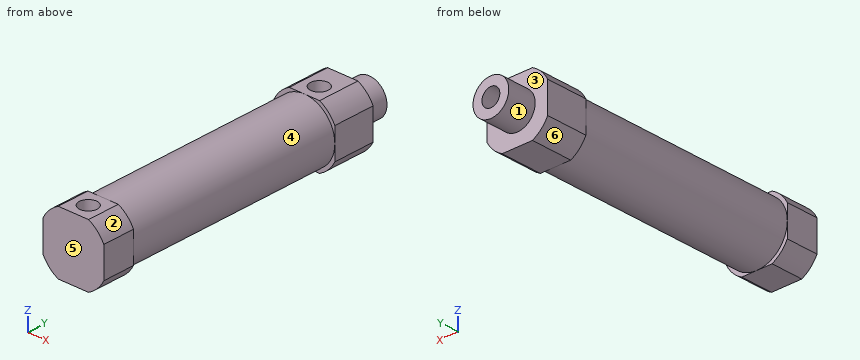
Autodesk Inventor part; units mm, degrees
ref_plane "YZ Plane" through (0, 0, 0) normal (1, 0, 0) x (0, 1, 0)
ref_plane "XZ Plane" through (0, 0, 0) normal (0, 1, 0) x (-1, 0, 0)
ref_plane "XY Plane" through (0, 0, 0) normal (0, 0, 1) x (1, 0, 0)
sketch "スケッチ1" plane through (0, 0, 0) normal (0, 1, 0) x (-1, 0, 0)
  circle A0 centre (0, 0) radius 8.5
  dimension "d0" = 17
extrude "押し出し1" add sketch "スケッチ1" along normal blind 61
sketch "スケッチ2" plane through (0, 61, 0) normal (0, 1, 0) x (1, 0, 0)
  circle A0 centre (0, 0) radius 9.5
  line L0 (8.5, -8.5) -> (-8.5, -8.5)
  line L1 (-8.5, -8.5) -> (-8.5, 8.5)
  line L2 (-8.5, 8.5) -> (8.5, 8.5)
  line L3 (8.5, 8.5) -> (8.5, -8.5)
  line L4 (8.5, -8.5) -> (-8.5, 8.5) construction
  line L5 (-8.5, -8.5) -> (8.5, 8.5) construction
  point P0 (8.5, -4.2426)
  point P1 (8.5, 4.2426)
  point P2 (4.2426, 8.5)
  point P3 (-4.2426, 8.5)
  point P4 (-8.5, 4.2426)
  point P5 (-8.5, -4.2426)
  point P6 (-4.2426, -8.5)
  point P7 (4.2426, -8.5)
  dimension "d3" = 19
  dimension "d4" = 17
  dimension "d5" = 17
extrude "押し出し2" add sketch "スケッチ2" along normal blind 11.6 contours L3 A0 L0 L1 L2
sketch "スケッチ3" plane through (0, 0, 0) normal (0, -1, 0) x (1, 0, 0)
  circle A0 centre (0, 0) radius 9.5
  line L0 (8.5, 8.5) -> (-8.5, 8.5)
  line L1 (-8.5, 8.5) -> (-8.5, -8.5)
  line L2 (-8.5, -8.5) -> (8.5, -8.5)
  line L3 (8.5, -8.5) -> (8.5, 8.5)
  line L4 (8.5, 8.5) -> (-8.5, -8.5) construction
  line L5 (-8.5, 8.5) -> (8.5, -8.5) construction
  point P0 (8.5, -4.2426)
  point P1 (8.5, 4.2426)
  point P2 (4.2426, 8.5)
  point P3 (-4.2426, 8.5)
  point P4 (-8.5, 4.2426)
  point P5 (-8.5, -4.2426)
  point P6 (-4.2426, -8.5)
  point P7 (4.2426, -8.5)
  dimension "d8" = 19
  dimension "d9" = 17
  dimension "d10" = 17
extrude "押し出し3" add sketch "スケッチ3" along normal blind 9 contours L3 A0 L2 L1 L0
sketch "スケッチ4" plane through (0, 72.6, 0) normal (0, 1, 0) x (1, 0, 0)
  circle A0 centre (0, 0) radius 5
  dimension "d13" = 10
extrude "押し出し4" add sketch "スケッチ4" along normal blind 8
thread "ねじ1"
sketch "スケッチ5" plane through (-4.2426, 61, 8.5) normal (0, 0, 1) x (1, 0, 0)
  line L0 (0, -61) -> (0, -70)
  line L1 (0, 0) -> (0, 11.6)
  line L2 (0, 11.6) -> (8.4853, 11.6)
  line L3 (0, 0) -> (4.2426, 0)
  point P0 (4.2426, -61)
  point P1 (4.2426, 4.5)
  point P2 (4.2426, -65.5)
  point P3 (0, -65.5)
  point P4 (0, 5.8)
  point P5 (4.2426, 11.6)
  dimension "d18" = 4.5
hole "穴1" at (0, 65.5, 8.5) at (0, -4.5, 8.5) direction (0, 0, -1) diameter 5 depth 10
thread "ねじ2"
thread "ねじ3"
sketch "スケッチ6" plane through (0, 80.6, 0) normal (0, 1, 0) x (1, 0, 0)
  circle A0 centre (0, 0) radius 5
hole "穴2" at (0, 80.6, 0) direction (0, -1, 0) diameter 5 depth 80.6
properties part number "KOGANEI_unkown_35_main" material "ステンレス鋼 440C"
For this review, take the finished solid that the model builds, in its own axes (mm). Face numbers are marked on the shaded views. A direction names the side the tool comes from. Give positions to 0.01 mm unless a question says otherwise; leave off trailing zeros. Loops run counter-clockwise (first coordinate to the right, second up) from the corner with the lowest first, then second, coordinate; pieces in that order, holes last.
Item 1: Draft analysis for pull direction Y (two halves, no side actions). For the marked faces 3, 4, 5 and 6, state which applies: +Y half, -Y half, draft (parallel to the pull), parting line (faces both ways), or undercut.
Item 2: Tool access review of the marked faces 1 and 2: name each direction out of +Z, -Z, +X, -X, +Y, -Y from which nothing blocks a thin tool from reaching the whole face with its end or side.
Item 3: Take a section at A-A, the plane y = 42.5. State the section outline as (x, z) points, and give its area (3 significant figures).
Item 4: Insertion check: pin 1 (10 mm diameter, centred on x = 1.5, z = -6, fed in from +Y); pin 2 (5 mm diameter, centred on y = 38, z = 6, fed in from -X); pin 3 (3 mm diameter, centred on x = 0, z = 0, fed in from +Y); pin 4 (8 mm diameter, centred on x = 5, y = 45, fed in from +Z). Each pin has a flat end and moves straight along its axis. Give the tip position at first contact, or say it passes through.
Item 5: Take a section at B-B, the plane z = -5.75. State the section outline as (x, y) points, and give its area (3 significant figures).
Item 6: For line 1 along Y through (x, z) = (0, 5.25); line 2 along X through (y, z) = (27.5, 0); line 3 along Y through (x, z) = (0, 3.5), list the stretches that pass through material, from the lowest coordinate up.
Calculated:
1. face 3: +Y half
1. face 4: undercut
1. face 5: -Y half
1. face 6: draft
2. face 1: +Y
2. face 2: +Z, +X, +Y, -Y
3. outline: circle Ø17 at (0, 0); hole circle Ø5 at (0, 0)
3. area: 207 mm2
4. pin 1: stops at y = 80.6
4. pin 2: stops at x = -7.75
4. pin 3: stops at y = 0
4. pin 4: stops at z = 8.44
5. outline: (-7.56, -9) - (7.56, -9) - (7.56, 0) - (6.26, 0) - (6.26, 61) - (7.56, 61) - (7.56, 72.6) - (-7.56, 72.6) - (-7.56, 61) - (-6.26, 61) - (-6.26, 0) - (-7.56, 0) - close
5. area: 1,080 mm2
6. line 1: y = -9 to -7, -2 to 63, 68 to 72.6
6. line 2: x = -8.5 to -2.5, 2.5 to 8.5
6. line 3: y = -9 to -7, -2 to 63, 68 to 80.6
